```python
from build123d import *

# Parameters (mm, degrees)
SKETCH1_W                              = 101.6
SKETCH1_H                              = 127
BOSS_EXTRUDE1_DEPTH                    = 12.7
CBORE_FOR_M5_HEX_HEAD_BOLT1_AT_2_COUNT = 2
CBORE_FOR_M5_HEX_HEAD_BOLT1_AT_2_PITCH = 18.0086
CBORE_FOR_M5_HEX_HEAD_BOLT1_AT_3_COUNT = 2
CBORE_FOR_M5_HEX_HEAD_BOLT1_AT_3_PITCH = 25.461925967
CBORE_FOR_M5_HEX_HEAD_BOLT1_AT_4_COUNT = 2
CBORE_FOR_M5_HEX_HEAD_BOLT1_AT_4_PITCH = 18
CBORE_FOR_M5_SHCS1_D                   = 5.5
CBORE_FOR_M5_SHCS1_CBORE_D             = 10
CBORE_FOR_M5_SHCS1_CBORE_DEPTH         = 5


with BuildPart() as part:
    # Sketch1 → Boss-Extrude1 (new body)
    with BuildSketch(Plane.XY):
        with Locations((50.8, 63.5)):
            Rectangle(SKETCH1_W, SKETCH1_H)
    extrude(amount=BOSS_EXTRUDE1_DEPTH)

    # Sketch8 → CBORE for M5 Hex Head Bolt1 (revolve, cut)
    with BuildSketch(Plane(origin=(41.7957, 72.5, 12.7), x_dir=(0, -1, 0), z_dir=(1, 0, 0))):
        Polygon((0, 0), (0, 12.7), (2.75, 12.7), (2.75, 3.58), (6.12, 3.58), (6.12, 0.025), (6.145, 0), align=None)
    cbore_for_m5_hex_head_bolt1 = revolve(axis=Axis((41.7957, 72.5, 19.05), (0, 0, -1)), mode=Mode.SUBTRACT)

    # CBORE for M5 Hex Head Bolt1 at 2: CBORE for M5 Hex Head Bolt1 ×2
    with Locations(*[(i * CBORE_FOR_M5_HEX_HEAD_BOLT1_AT_2_PITCH, 0, 0) for i in range(1, CBORE_FOR_M5_HEX_HEAD_BOLT1_AT_2_COUNT)]):
        add(cbore_for_m5_hex_head_bolt1, mode=Mode.SUBTRACT)

    # CBORE for M5 Hex Head Bolt1 at 3: CBORE for M5 Hex Head Bolt1 ×2
    with Locations(*[Vector(0.7072756406246394, -0.7069378814146302, 0) * (i * CBORE_FOR_M5_HEX_HEAD_BOLT1_AT_3_PITCH) for i in range(1, CBORE_FOR_M5_HEX_HEAD_BOLT1_AT_3_COUNT)]):
        add(cbore_for_m5_hex_head_bolt1, mode=Mode.SUBTRACT)

    # CBORE for M5 Hex Head Bolt1 at 4: CBORE for M5 Hex Head Bolt1 ×2
    with Locations(*[(0, -i * CBORE_FOR_M5_HEX_HEAD_BOLT1_AT_4_PITCH, 0) for i in range(1, CBORE_FOR_M5_HEX_HEAD_BOLT1_AT_4_COUNT)]):
        add(cbore_for_m5_hex_head_bolt1, mode=Mode.SUBTRACT)

    # CBORE for M5 SHCS1 (through all)
    with Locations(Plane.XY.offset(12.7)):
        with Locations((12.7, 114.3), (88.9, 114.3), (88.9, 12.7), (12.7, 12.7)):
            CounterBoreHole(CBORE_FOR_M5_SHCS1_D / 2, CBORE_FOR_M5_SHCS1_CBORE_D / 2, CBORE_FOR_M5_SHCS1_CBORE_DEPTH)


solid = part.part
```
Geometry check sheet. Reference: the model listing, model coordinates, mm. A direction names the side the tool comes from. Give positions to 0.01 mm unless a question says otherwise; leave off trailing zeros. Order: outer loops, then holes, each group sorted by start corner. A loop starts at its lowest first (then second) coordinate and runs counter-clockwise, first axis right, second up.
1. Gauge pin test, flat ends, axial feed: pin 1 Ø9 at (x, y) = (88.9, 114.3) entering from +Z; pin 2 Ø10 at (x, y) = (41.8, 54.5) entering from +Z; pin 3 Ø3.5 at (x, y) = (41.8, 54.5) entering from -Z. Record the tip position at first contact, or that the pin passes through.
2. Thickness scan on L1, parallel to Y at x = 59.5, z = 8.75; L2, parallel to X at y = 54.5, z = 10.65; L3, parallel to Y at x = 88.9, z = 11.4. Record the ranges inside material, lowest first.
3. Release check for a two-part mould opening along Y. For faces 3 (the face through (101.6, 63, 6)), 4 (the face through (83.905, 12.92, 10.235)), 5 (the face through (11.62, 109.42, 10.24)), 6 (the face through (50, 0, 6)) record: pulls with the +Y half, pulls with the -Y half, needs draft (parallel to the pull), parting line crosses it, or undercut.
4. Access from +Z, -Z, +X, -X, +Y, -Y to the whole of each face (thin tool, end or side, straight path). Record for faces 1 (the face through (86.28, 13.53, 3.8)), 2 (the face through (15, 112, 7.7)).
5. Section check B-B, the plane x = 88.9. Enter the section's corners in (y, z), and give its area (3 significant figures).
6. Section check C-C, the plane y = 114.3. Enter the section's corners in (x, z).
7. Section check A-A, the plane y = 54.5. Enter the section's corners in (x, z) (3 decimals), and give its area (3 significant figures).
Values follow:
1. pin 1: stops at z = 7.7
1. pin 2: stops at z = 9.12
1. pin 3: passes through
2. L1: y = 0 to 51.77, 57.23 to 69.77, 75.23 to 127
2. L2: x = 0 to 35.68, 47.92 to 53.68, 65.92 to 101.6
2. L3: y = 0 to 7.7, 17.7 to 109.3, 119.3 to 127
3. face 3: needs draft
3. face 4: undercut
3. face 5: undercut
3. face 6: pulls with the -Y half
4. face 1: +Z, -Z
4. face 2: +Z
5. outline: (0, 0) - (9.95, 0) - (9.95, 7.7) - (7.7, 7.7) - (7.7, 12.7) - (0, 12.7) - close; (15.45, 0) - (111.55, 0) - (111.55, 7.7) - (109.3, 7.7) - (109.3, 12.7) - (17.7, 12.7) - (17.7, 7.7) - (15.45, 7.7) - close; (117.05, 0) - (127, 0) - (127, 12.7) - (119.3, 12.7) - (119.3, 7.7) - (117.05, 7.7) - close
5. area: 1,430 mm2
6. outline: (0, 0) - (9.95, 0) - (9.95, 7.7) - (7.7, 7.7) - (7.7, 12.7) - (0, 12.7) - close; (15.45, 0) - (86.15, 0) - (86.15, 7.7) - (83.9, 7.7) - (83.9, 12.7) - (17.7, 12.7) - (17.7, 7.7) - (15.45, 7.7) - close; (91.65, 0) - (101.6, 0) - (101.6, 12.7) - (93.9, 12.7) - (93.9, 7.7) - (91.65, 7.7) - close
7. outline: (0, 0) - (39.046, 0) - (39.046, 9.12) - (35.676, 9.12) - (35.676, 12.675) - (35.651, 12.7) - (0, 12.7) - close; (44.546, 0) - (57.054, 0) - (57.054, 9.12) - (53.684, 9.12) - (53.684, 12.675) - (53.659, 12.7) - (47.941, 12.7) - (47.916, 12.675) - (47.916, 9.12) - (44.546, 9.12) - close; (62.554, 0) - (101.6, 0) - (101.6, 12.7) - (65.949, 12.7) - (65.924, 12.675) - (65.924, 9.12) - (62.554, 9.12) - close
7. area: 1,100 mm2
